```python
from build123d import *

# Parameters (mm, degrees)
SKETCH_W      = 40
SKETCH_H      = 70
SKETCH_R      = 5.5
SKETCH_W_2    = 16
SKETCH_H_2    = 21
PAD_DEPTH     = 2
SKETCH001_W   = 5.6
SKETCH001_H   = 5.6
SKETCH001_W_2 = 16
SKETCH001_H_2 = 21
PAD001_DEPTH  = 6.5
SKETCH002_W   = 16
SKETCH002_H   = 1
SKETCH002_W_2 = 4.092667
POCKET_DEPTH  = 1.5
SKETCH003_R   = 1.625
PAD002_DEPTH  = 2.5


with BuildPart() as part:
    # Sketch → Pad (new body)
    with BuildSketch(Plane.XY):
        Rectangle(SKETCH_W, SKETCH_H)
        with Locations((0, 23)):
            Circle(SKETCH_R, mode=Mode.SUBTRACT)
        Rectangle(SKETCH_W_2, SKETCH_H_2, mode=Mode.SUBTRACT)
    extrude(amount=PAD_DEPTH)

    # Sketch001 (on Face11 of Pad) → Pad001 (join)
    with BuildSketch(Plane.XY.offset(2)):
        with Locations((-8.5, -18.5)):
            Rectangle(SKETCH001_W, SKETCH001_H)
        with Locations((8.5, -18.5)):
            Rectangle(SKETCH001_W, SKETCH001_H)
        with BuildLine():
            Line((-8, -11.5), (8, -11.5))
            ThreePointArc((9, -10.5), (8.7071067812, -11.2071067812), (8, -11.5))
            Line((9, -10.5), (9, 10.5))
            ThreePointArc((8, 11.5), (8.7071067812, 11.2071067812), (9, 10.5))
            Line((8, 11.5), (-8, 11.5))
            ThreePointArc((-9, 10.5), (-8.7071067812, 11.2071067812), (-8, 11.5))
            Line((-9, 10.5), (-9, -10.5))
            ThreePointArc((-8, -11.5), (-8.7071067812, -11.2071067812), (-9, -10.5))
        make_face()
        Rectangle(SKETCH001_W_2, SKETCH001_H_2, mode=Mode.SUBTRACT)
    extrude(amount=PAD001_DEPTH)

    # Sketch002 (on Face34 of Pad001) → Pocket (cut)
    with BuildSketch(Plane.XY.offset(8.5)):
        with Locations((0, 11)):
            Rectangle(SKETCH002_W, SKETCH002_H)
        with Locations((6.9536665, -11)):
            Rectangle(SKETCH002_W_2, SKETCH002_H)
    extrude(amount=-POCKET_DEPTH, mode=Mode.SUBTRACT)

    # Sketch003 (on Face32 of Pocket) → Pad002 (join)
    with BuildSketch(Plane.XY.offset(8.5)):
        with Locations((-8.5, -18.5)):
            Circle(SKETCH003_R)
        with Locations((8.5, -18.5)):
            Circle(SKETCH003_R)
    extrude(amount=PAD002_DEPTH)


solid = part.part
```
Could you check a few things on this model? Use its own coordinates, in mm. A direction names the side the tool comes from. Coordinates: 2 decimals unless noted, no trailing zeros. Loops run counter-clockwise (first coordinate to the right, second up) from the corner with the lowest first, then second, coordinate; pieces in that order, holes last. Notation, with made-up numbers: M 75.25,-38.75 L 106.25,-38.75 A38 cw 106.25,0.25 Z; hole C -22.75,-26 d10. An arc over 180 degrees is marked long. Put each result on its own line as item: value. Start each with the question number.
(1) Will these pins go through, and if not, where does the flat tip stop? P1, Ø4, axis at x = -5.5, y = 3.5, coming from the +Z side; P2, Ø3, axis at y = -3.5, z = 8, coming from the +X side; P3, Ø0.8, axis at x = -0.5, y = 11, coming from the +Z side; P4, Ø4.5, axis at y = -19, z = 6, coming from the +X side.
(2) Suppose I cut it at A-A on z = 3.5. Please give me the cut outline in (x, y), then the cut area to 3 significant figures.
(3) Suppose I cut it at B-B on x = 0. Please give me the cut outline in (y, z).
(4) For faces 4 (the face through (8.148, -20.086, 9.732)), 5 (the face through (0, -10.5, 4)), 6 (the face through (-11.3, -19, 5)), which set-ups out of +Z, -Z, +X, -X, +Y, -Y let a thin tool reach every point of the face, with its end or its side?
(5) Suppose I cut it at C-C on y = -3.5. Please give me the cut outline in (x, z).
(6) I need wall thicknesses on line 1 (Y direction, x = 0, z = 0.65); line 2 (Z direction, x = -11, y = -5); line 3 (Y direction, x = -2.5, z = 1.75). Which ranges of each line are inside material? Lowest first, please. Write a range as from..to.
(7) Suppose I cut it at D-D on y = -18.5. Please give me the cut outline in (x, z) (3 decimals).
(8) Thinking about a two-plate mould opening in X: for faces 1 (the face through (-8.852, -20.086, 9.732)), 2 (the face through (11.3, -19, 5)), 3 (the face through (8, -18, 11)), which applies, pulls with the +X half, pulls with the -X half, needs draft (parallel to the pull), parting line crosses it, or undercut?
Solutions:
1. P1: passes through
1. P2: stops at x = 9
1. P3: stops at z = 7
1. P4: stops at x = 11.3
2. outline: M -11.3,-21.3 L -5.7,-21.3 L -5.7,-15.7 L -11.3,-15.7 Z; M -9,-10.5 A1 ccw -8,-11.5 L 8,-11.5 A1 ccw 9,-10.5 L 9,10.5 A1 ccw 8,11.5 L -8,11.5 A1 ccw -9,10.5 Z; M 5.7,-21.3 L 11.3,-21.3 L 11.3,-15.7 L 5.7,-15.7 Z; hole M -8,-10.5 L 8,-10.5 L 8,10.5 L -8,10.5 Z
2. area: 140 mm2
3. outline: M -35,0 L -10.5,0 L -10.5,8.5 L -11.5,8.5 L -11.5,2 L -35,2 Z; M 10.5,0 L 17.5,0 L 17.5,2 L 11.5,2 L 11.5,7 L 10.5,7 Z; M 28.5,0 L 35,0 L 35,2 L 28.5,2 Z
4. face 4: +Z
4. face 5: +Z, -Z
4. face 6: +Z, -X, +Y, -Y
5. outline: M -20,0 L -8,0 L -8,8.5 L -9,8.5 L -9,2 L -20,2 Z; M 8,0 L 20,0 L 20,2 L 9,2 L 9,8.5 L 8,8.5 Z
6. line 1: y = -35..-10.5, 10.5..17.5, 28.5..35
6. line 2: z = 0..2
6. line 3: y = -35..-10.5, 10.5..18.1, 27.9..35
7. outline: M -20,0 L 20,0 L 20,2 L 11.3,2 L 11.3,8.5 L 10.125,8.5 L 10.125,11 L 6.875,11 L 6.875,8.5 L 5.7,8.5 L 5.7,2 L -5.7,2 L -5.7,8.5 L -6.875,8.5 L -6.875,11 L -10.125,11 L -10.125,8.5 L -11.3,8.5 L -11.3,2 L -20,2 Z
8. face 1: undercut
8. face 2: pulls with the +X half
8. face 3: needs draft
